Verification items for the finished model (mm, model axes). Face numbers are marked on the shaded views. A direction names the side the tool comes from. Give positions to 0.01 mm unless a question says otherwise; leave off trailing zeros. Write each loop counter-clockwise with the first axis right and the second up, starting at its lowest first coordinate (ties: lowest second). Pieces come first, ordered by that corner, then holes. Notation, with made-up numbers: (9, -5.75) - (64, -5.75) arc R16 ccw to (64, 12.25) - close; hole circle Ø2 at (7.5, 6). An arc over 180 degrees is marked (long way). Answer as a JSON object with one key per item and string values. Group by question number.
Item 1: Sectioned sample at C-C, the plane z = -9. Record the boundary of the cut face in (x, y).
Item 2: Draft check along X on the marked faces 1, 2, 3 and 4. Enter one of: +X half, -X half, draft (parallel to the pull), parting line (faces both ways), or undercut.
Item 3: Sectioned sample at A-A, the plane x = 0. Record the boundary of the cut face in (y, z), and give its area (3 significant figures).
Item 4: Tool access check on the marked faces 5, 6, 7 and 8. Record the directions out of +Z, -Z, +X, -X, +Y, -Y that give a thin tool (end or side, any length) a straight path to the whole face; none if there is none.
Item 5: Sectioned sample at B-B, the plane y = -34. Record the boundary of the cut face in (x, z) (1 decimal).
Item 6: Sectioned sample at D-D, the plane x = 8.5. Record the boundary of the cut face in (y, z), and give its area (3 significant figures).
Item 7: Go/stop test with flat-tipped pins: pin 1 (12 mm diameter, centred on y = -46, z = 4, fed in from +X); pin 2 (5 mm diameter, centred on x = -18.5, y = -29.5, fed in from -Z); pin 3 (8 mm diameter, centred on x = 10.5, y = -18.5, fed in from -Z). Record where each tip stops, or that it passes through.
Item 8: Scan lines: line 1 along X through (y, z) = (-8, -3); line 2 along X through (y, z) = (-62, 1); line 3 along Y through (x, z) = (7, 3). Record each from-to range of solid material in increasing order. Write a range as [from, to].
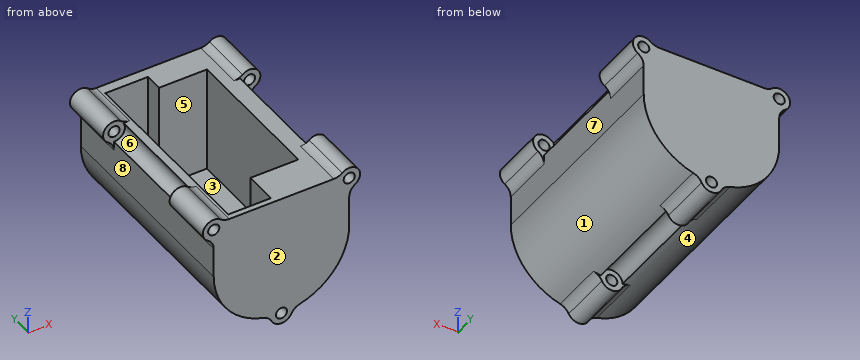
```python
from build123d import *

# Parameters (mm, degrees)
SKETCH1_R               = 38.1
BULKHEAD_BODY_DEPTH     = 12.7
SKETCH2_R               = 1.5875
CUT_EXTRUDE1_DEPTH      = 12.7
BOSS_EXTRUDE1_OUTLINE_R = 2.0875
BOSS_EXTRUDE1_DEPTH     = 80
CUT_EXTRUDE4_DEPTH      = 20
CUT_EXTRUDE4_DEPTH_BACK = 20
SKETCH5_R               = 4.0875
FILLET1_START           = -80
FILLET1_DEPTH           = 20
FILLET1_START_2         = -20
FILLET1_2_DEPTH         = 20
CUT_EXTRUDE5_DEPTH      = 34
SKETCH4_5_W             = 18
SKETCH4_5_H             = 55
CUT_EXTRUDE6_DEPTH      = 40


with BuildPart() as part:
    # Sketch1 → Bulkhead Body (new body)
    with BuildSketch(Plane(origin=(0, 0, 0), x_dir=(1, 0, 0), z_dir=(0, 1, 0))):
        with Locations(Location((0, 0, 0), (0, 0, 270))):
            Circle(SKETCH1_R)
    extrude(amount=BULKHEAD_BODY_DEPTH)

    # Sketch2 → Cut-Extrude1 (cut)
    with BuildSketch(Plane(origin=(0, 12.7, 0), x_dir=(1, 0, 0), z_dir=(0, 1, 0))):
        with Locations(Location((0, 29.337, 0), (0, 0, 270))):
            Circle(SKETCH2_R)
        with Locations(Location((25.406587271, -14.5685, 0), (0, 0, 270))):
            Circle(SKETCH2_R)
        with Locations(Location((-25.31998473, -14.6185, 0), (0, 0, 270))):
            Circle(SKETCH2_R)
    extrude(amount=-CUT_EXTRUDE1_DEPTH, mode=Mode.SUBTRACT)


with BuildPart() as body_2:
    # Boss-Extrude1: read off the stored shape, not the designer's step
    # Boss-Extrude1 outline → Boss-Extrude1 (new body)
    with BuildSketch(Plane(origin=(0, 0, 0), x_dir=(-1, 0, 0), z_dir=(0, -1, 0))):
        with BuildLine():
            ThreePointArc((-4.078497939, 29.065871225), (-19.338013085, 20.664924444), (-25.406587271, 4.337))
            Line((-25.406587271, 4.337), (-25.406587271, -10.581))
            ThreePointArc((-25.406587271, -10.581), (-28.933813961, -16.734009168), (-21.841807299, -16.6685))
            Line((-21.841807299, -16.6685), (21.841807299, -16.6685))
            ThreePointArc((21.841807299, -16.6685), (28.933813961, -16.734009168), (25.406587271, -10.581))
            Line((25.406587271, -10.581), (25.406587271, 4.337))
            ThreePointArc((25.406587271, 4.337), (19.338013085, 20.664924444), (4.078497939, 29.065871225))
            ThreePointArc((4.078497939, 29.065871225), (0, 33.4245), (-4.078497939, 29.065871225))
        make_face()
        with Locations((-25.406587271, -14.6685)):
            Circle(BOSS_EXTRUDE1_OUTLINE_R, mode=Mode.SUBTRACT)
        with Locations((25.406587271, -14.6685)):
            Circle(BOSS_EXTRUDE1_OUTLINE_R, mode=Mode.SUBTRACT)
        with Locations((0, 29.337)):
            Circle(BOSS_EXTRUDE1_OUTLINE_R, mode=Mode.SUBTRACT)
    extrude(amount=BOSS_EXTRUDE1_DEPTH)

    # Sketch5 → Cut-Extrude4 (cut, two sides: drawn at the far end of the back side and taken through both)
    with BuildSketch(Plane(origin=(0, -40, 0), x_dir=(-1, 0, 0), z_dir=(0, -1, 0)).offset(-CUT_EXTRUDE4_DEPTH_BACK)):
        with Locations((25.406587271, -14.6685)):
            Circle(SKETCH5_R)
        with Locations((-25.406587271, -14.6685)):
            Circle(SKETCH5_R)
        with Locations((0, 29.337)):
            Circle(SKETCH5_R)
    extrude(amount=CUT_EXTRUDE4_DEPTH + CUT_EXTRUDE4_DEPTH_BACK, mode=Mode.SUBTRACT)

    # Fillet1: read off the stored shape, not the designer's step
    # Fillet1 outline → Fillet1 (add)
    with BuildSketch(Plane(origin=(0, 0, 0), x_dir=(1, 0, 0), z_dir=(0, 1, 0)).offset(FILLET1_START)):
        with BuildLine():
            ThreePointArc((-4.078497939, 29.065871225), (-4.011334199, 30.122400658), (-3.67508636, 31.126244671))
            ThreePointArc((-3.67508636, 31.126244671), (-4.988887184, 29.457894165), (-6.876601915, 28.485269307))
            ThreePointArc((-6.876601915, 28.485269307), (-5.485852661, 28.815583764), (-4.078497939, 29.065871225))
        make_face()
        with BuildLine():
            ThreePointArc((6.876601915, 28.485269307), (4.988887184, 29.457894165), (3.67508636, 31.126244671))
            ThreePointArc((3.67508636, 31.126244671), (4.011334199, 30.122400658), (4.078497939, 29.065871225))
            ThreePointArc((4.078497939, 29.065871225), (5.485852661, 28.815583764), (6.876601915, 28.485269307))
        make_face()
        with BuildLine():
            Line((-25.406587271, -10.581), (-25.406587271, -7.080176321))
            ThreePointArc((-25.406587271, -7.080176321), (-26.0045901, -9.451340784), (-27.655555634, -11.255320024))
            ThreePointArc((-27.655555634, -11.255320024), (-26.580530007, -10.753207584), (-25.406587271, -10.581))
        make_face()
        with BuildLine():
            ThreePointArc((27.655555634, -11.255320024), (26.0045901, -9.451340784), (25.406587271, -7.080176321))
            Line((25.406587271, -7.080176321), (25.406587271, -10.581))
            ThreePointArc((25.406587271, -10.581), (26.580530007, -10.753207584), (27.655555634, -11.255320024))
        make_face()
        with BuildLine():
            ThreePointArc((-21.841807299, -16.6685), (-22.267923157, -17.286981206), (-22.80000844, -17.817055708))
            ThreePointArc((-22.80000844, -17.817055708), (-21.306050221, -16.964394269), (-19.611532806, -16.6685))
            Line((-19.611532806, -16.6685), (-21.841807299, -16.6685))
        make_face()
        with BuildLine():
            ThreePointArc((19.611532806, -16.6685), (21.306050221, -16.964394269), (22.80000844, -17.817055708))
            ThreePointArc((22.80000844, -17.817055708), (22.267923157, -17.286981206), (21.841807299, -16.6685))
            Line((21.841807299, -16.6685), (19.611532806, -16.6685))
        make_face()
    extrude(amount=FILLET1_DEPTH)

    # Fillet1 2 outline → Fillet1 2 (add)
    with BuildSketch(Plane(origin=(0, 0, 0), x_dir=(1, 0, 0), z_dir=(0, 1, 0)).offset(FILLET1_START_2)):
        with BuildLine():
            ThreePointArc((-4.078497939, 29.065871225), (-4.011334199, 30.122400658), (-3.67508636, 31.126244671))
            ThreePointArc((-3.67508636, 31.126244671), (-4.988887184, 29.457894165), (-6.876601915, 28.485269307))
            ThreePointArc((-6.876601915, 28.485269307), (-5.485852661, 28.815583764), (-4.078497939, 29.065871225))
        make_face()
        with BuildLine():
            ThreePointArc((6.876601915, 28.485269307), (4.988887184, 29.457894165), (3.67508636, 31.126244671))
            ThreePointArc((3.67508636, 31.126244671), (4.011334199, 30.122400658), (4.078497939, 29.065871225))
            ThreePointArc((4.078497939, 29.065871225), (5.485852661, 28.815583764), (6.876601915, 28.485269307))
        make_face()
        with BuildLine():
            Line((-25.406587271, -10.581), (-25.406587271, -7.080176321))
            ThreePointArc((-25.406587271, -7.080176321), (-26.0045901, -9.451340784), (-27.655555634, -11.255320024))
            ThreePointArc((-27.655555634, -11.255320024), (-26.580530007, -10.753207584), (-25.406587271, -10.581))
        make_face()
        with BuildLine():
            ThreePointArc((27.655555634, -11.255320024), (26.0045901, -9.451340784), (25.406587271, -7.080176321))
            Line((25.406587271, -7.080176321), (25.406587271, -10.581))
            ThreePointArc((25.406587271, -10.581), (26.580530007, -10.753207584), (27.655555634, -11.255320024))
        make_face()
        with BuildLine():
            ThreePointArc((-21.841807299, -16.6685), (-22.267923157, -17.286981206), (-22.80000844, -17.817055708))
            ThreePointArc((-22.80000844, -17.817055708), (-21.306050221, -16.964394269), (-19.611532806, -16.6685))
            Line((-19.611532806, -16.6685), (-21.841807299, -16.6685))
        make_face()
        with BuildLine():
            ThreePointArc((19.611532806, -16.6685), (21.306050221, -16.964394269), (22.80000844, -17.817055708))
            ThreePointArc((22.80000844, -17.817055708), (22.267923157, -17.286981206), (21.841807299, -16.6685))
            Line((21.841807299, -16.6685), (19.611532806, -16.6685))
        make_face()
    extrude(amount=FILLET1_2_DEPTH)

    # Sketch4 → Cut-Extrude5 (cut)
    with BuildSketch(Plane.XY.offset(16.6685)):
        Polygon((-2.620203368, -65.485753458), (-2.620203368, -10.485753458), (-2.620203368, -3.842418919), (-18.620203368, -3.842418919), (-18.620203368, -77.842418919), (-2.620203368, -77.842418919), align=None)
    extrude(amount=-CUT_EXTRUDE5_DEPTH, mode=Mode.SUBTRACT)

    # Sketch4<5> → Cut-Extrude6 (cut)
    with BuildSketch(Plane.XY.offset(16.6685)):
        with Locations((6.379796632, -37.985753458)):
            Rectangle(SKETCH4_5_W, SKETCH4_5_H)
    extrude(amount=-CUT_EXTRUDE6_DEPTH, mode=Mode.SUBTRACT)


solid = body_2.part
```
Geometry check:
{
 "1": {"outline": "(-24.97, -80) - (24.97, -80) - (24.97, 0) - (-24.97, 0) - close; hole (-18.62, -77.84) - (-2.62, -77.84) - (-2.62, -65.49) - (15.38, -65.49) - (15.38, -10.49) - (-2.62, -10.49) - (-2.62, -3.84) - (-18.62, -3.84) - close"},
 "2": {"face 1": "+X half", "face 2": "draft", "face 3": "undercut", "face 4": "-X half"},
 "3": {"outline": "(-80, -33.42) - (-60, -33.42) - (-60, -31.42) - (-80, -31.42) - close; (-80, -27.25) - (-60, -27.25) - (-60, -25.25) - (-20, -25.25) - (-20, -27.25) - (0, -27.25) - (0, 16.67) - (-10.49, 16.67) - (-10.49, -23.33) - (-65.49, -23.33) - (-65.49, 16.67) - (-80, 16.67) - close; (-20, -33.42) - (0, -33.42) - (0, -31.42) - (-20, -31.42) - close", "area": "1,310 mm^2"},
 "4": {"face 5": "+Z", "face 6": "-X", "face 7": "-Z, +X", "face 8": "-Z, -X"},
 "5": {"outline": "(-25.4, -4.3) arc R25 ccw to (-4.1, -29.1) arc R4.1 cw to (4.1, -29.1) arc R25 ccw to (25.4, -4.3) - (25.4, 10.6) arc R4.1 cw to (21.8, 16.7) - (15.4, 16.7) - (15.4, -23.3) - (-2.6, -23.3) - (-2.6, -17.3) - (-18.6, -17.3) - (-18.6, 16.7) - (-21.8, 16.7) arc R4.1 cw to (-25.4, 10.6) - close"},
 "6": {"outline": "(-80, -27.99) - (0, -27.99) - (0, 16.67) - (-10.49, 16.67) - (-10.49, -23.33) - (-65.49, -23.33) - (-65.49, 16.67) - (-80, 16.67) - close", "area": "1,370 mm^2"},
 "7": {"pin 1": "x = 25.41", "pin 2": "z = -23.88", "pin 3": "z = -28.6"},
 "8": {"line 1": "[-25.41, -18.62], [-2.62, 25.41]", "line 2": "[-25.41, -18.62], [15.38, 25.41]", "line 3": "[-80, -65.49], [-10.49, 0]"}
}
